Autodesk Inventor part; units mm, degrees
ref_plane "YZ Plane" through (0, 0, 0) normal (1, 0, 0) x (0, 1, 0)
ref_plane "XZ Plane" through (0, 0, 0) normal (0, 1, 0) x (-1, 0, 0)
ref_plane "XY Plane" through (0, 0, 0) normal (0, 0, 1) x (1, 0, 0)
sketch "Sketch1" plane through (0, 0, 0) normal (0, 0, 1) x (1, 0, 0)
  circle A0 centre (0, 0) radius 8.7
  arc A1 (11.985896, 6.635383) -> (-11.985896, 6.635383) centre (0, 0) ccw
  line L0 (0, 52.910691) -> (0, -52.910691) construction
  line L1 (-45, -53) -> (45, -53)
  line L2 (-45, -53) -> (-11.985896, 6.635383)
  line L3 (45, -53) -> (11.985896, 6.635383)
  line L4 (12.533127, -15) -> (23.881912, -35.5)
  line L5 (23.881912, -35.5) -> (-23.881912, -35.5)
  line L6 (-12.533127, -15) -> (12.533127, -15)
  line L7 (-23.881912, -35.5) -> (-12.533127, -15)
  circle A2 centre (0, 0) radius 8.65
  dimension "d0" = 5
  dimension "d1" = 53
  dimension "d2" = 90
  dimension "d3" = 45
  dimension "d12" = 17.5
  dimension "d13" = 15
  dimension "d15" = 10
  dimension "d16" = 10
  dimension "d41" = 17.3
sketch "Sketch1 outline for Extrusion1" plane through (0, 0, 0) normal (0, 0, 1) x (1, 0, 0)
  line L0 (-45, -53) -> (45, -53)
  line L1 (45, -53) -> (11.985896, 6.635383)
  arc A0 (11.985896, 6.635383) -> (-11.985896, 6.635383) centre (0, 0) ccw
  line L2 (-11.985896, 6.635383) -> (-45, -53)
  line L3 (12.533127, -15) -> (23.881912, -35.5)
  line L4 (23.881912, -35.5) -> (-23.881912, -35.5)
  line L5 (-23.881912, -35.5) -> (-12.533127, -15)
  line L6 (-12.533127, -15) -> (12.533127, -15)
  circle A1 centre (0, 0) radius 8.65
extrude "Extrusion1" add sketch "Sketch1 outline for Extrusion1" along normal blind 5
sketch "Sketch2" plane through (0, 0, 5) normal (0, 0, 1) x (1, 0, 0)
  line L0 (45, -53) -> (11.985896, 6.635383)
  arc A0 (11.985896, 6.635383) -> (-11.985896, 6.635383) centre (0, 0) ccw
  line L1 (-11.985896, 6.635383) -> (-45, -53)
  line L2 (-45, -53) -> (45, -53)
  line L3 (12.533127, -15) -> (23.881912, -35.5)
  line L4 (23.881912, -35.5) -> (-23.881912, -35.5)
  line L5 (-23.881912, -35.5) -> (-12.533127, -15)
  line L6 (-12.533127, -15) -> (12.533127, -15)
  line L7 (39.910172, -50) -> (9.361247, 5.182379)
  arc A1 (9.361247, 5.182379) -> (-9.361247, 5.182379) centre (0, 0) ccw
  line L8 (-9.361247, 5.182379) -> (-39.910172, -50)
  line L9 (-39.910172, -50) -> (39.910172, -50)
  line L10 (-14.301359, -12) -> (-28.97174, -38.5)
  line L11 (-28.97174, -38.5) -> (28.97174, -38.5)
  line L12 (28.97174, -38.5) -> (14.301359, -12)
  line L13 (14.301359, -12) -> (-14.301359, -12)
  circle A2 centre (0, 0) radius 8.65
  point P0 (0, 0)
  point P1 (-11.653536, 1.041678)
  point P2 (11.653536, 1.041678)
  dimension "d19" = 3
  dimension "d20" = 3
  dimension "d42" = 17.3
extrude "Extrusion2" add sketch "Sketch2" along normal blind 5 contours L2 L1 A0 L0 | L9 L8 A1 L7 | L13 L12 L11 L10
sketch "Sketch3" plane through (-45, -53, 0) normal (0, -1, 0) x (1, 0, 0)
  line L0 (45, 0) -> (45, 10) construction
  line L1 (32.466873, 10) -> (57.533127, 10) construction
  line L2 (0, 0) -> (0, 10) construction
  line L3 (0, 5) -> (90, 5) construction
  line L4 (90, 0) -> (90, 10) construction
  line L5 (33.3, 5) -> (56.7, 5) construction
  circle A0 centre (45, 5) radius 8.65
  circle A1 centre (45, 5) radius 3.5
  circle A2 centre (45, 5) radius 4.5
  circle A3 centre (77.5, 5) radius 1.7
  circle A4 centre (65, 5) radius 1.7
  circle A5 centre (12.5, 5) radius 1.7
  circle A6 centre (25, 5) radius 1.7
  point P0 (56.653536, 5)
  point P1 (33.346464, 5)
  dimension "d24" = 17.3
  dimension "d25" = 7
  dimension "d32" = 9
  dimension "d35" = 3.4
  dimension "d36" = 12.5
  dimension "d37" = 3.4
  dimension "d38" = 12.5
extrude "Extrusion3" cut sketch "Sketch3" against normal blind 5 contours A0 | A2
extrude "Extrusion4" cut sketch "Sketch3" against normal blind 43 contours A1
extrude "Extrusion5" cut sketch "Sketch3" against normal up to surface (5 mm away) from surface at -38 contours A0 | A2
extrude "Extrusion6" cut sketch "Sketch3" against normal blind 6 from surface at -38 contours A1 | A2
extrude "Extrusion7" cut sketch "Sketch3" against normal blind 13 contours A3 | A4 | A5 | A6
properties part number "96mmWheelBracket_3DPrint"
For this review, take the finished solid that the model builds, in its own axes (mm). A direction names the side the tool comes from. Coordinates: 2 decimals unless noted, no trailing zeros. Order: outer loops, then holes, each group sorted by start corner. A loop starts at its lowest first (then second) coordinate and runs counter-clockwise, first axis right, second up. Notation, with made-up numbers: (-6, 66) - (47, 66) arc R28 cw to (47, 98) - close; hole circle Ø2 at (18.5, -35.75). An arc over 180 degrees is marked (long way). Answer as a JSON object with one key per item and string values. Group by question number.
1. Clearance check with flat-ended pins moving along their axes: P1, Ø4, axis at x = 9, z = 4, coming from the +Y side; P2, Ø3, axis at x = -2.5, z = 3, coming from the -Y side; P3, Ø3, axis at x = -5.5, z = 3, coming from the +Y side; P4, Ø12, axis at x = 28.5, y = -7.5, coming from the -Z side. State where each tip first meets the part, or that it passes through.
2. We need section B-B on x = -14.5. State the section outline as (y, z) points, then the cut area to 3 significant figures.
3. The part is to be moulded in two halves that separate along X. For faces 1 (the flat face through (26, -53, 5)), 2 (the flat face through (4, -48, 5)), 3 (the cylindrical face through (21.57, -46.59, 4.35)), say which applies: pulls with the +X half, pulls with the -X half, needs draft (parallel to the pull), parting line crosses it, or undercut.
4. We need section A-A on y = -2. State the section outline as (x, z) points.
5. For faces 4 (the cylindrical face through (-18.43, -46.59, 4.35)), 5 (the flat face through (-26, -53, 5)), 6 (the flat face through (10, -15, 5)), 7 (the cylindrical face through (8.65, -12.54, 4.93)), list the 3-axis set-ups (+Z, -Z, +X, -X, +Y, -Y) from which the entire face can be reached by the end or side of a thin tool; tool diameter is ignored.
6. We need section C-C on x = 0. State the section outline as (y, z) points.
7. For probe 1 along Z at (x, y) = (0, -9.75); probe 2 along Z at (x, y) = (32.5, -42.5); probe 3 along Y at (x, z) = (0.5, 4), list the stretches that pass through material, from the lowest coordinate up.
8. We need section D-D on y = -39. State the section outline as (x, z) points, then the cut area to 3 significant figures.
Final values:
{
 "1": {"P1": "y = 11.78", "P2": "y = -48", "P3": "y = 13.1", "P4": "through"},
 "2": {"outline": "(-53, 0) - (-35.5, 0) - (-35.5, 10) - (-53, 10) - close; (-18.55, 0) - (2.09, 0) - (2.09, 10) - (-18.55, 10) - close", "area": "381 mm²"},
 "3": {"face 1": "needs draft", "face 2": "undercut", "face 3": "undercut"},
 "4": {"outline": "(-16.77, 0) - (-8.42, 0) - (-8.42, 10) - (-16.77, 10) - close; (8.42, 0) - (16.77, 0) - (16.77, 10) - (8.42, 10) - close"},
 "5": {"face 4": "-Y", "face 5": "+Z, -Z, +X, -X, -Y", "face 6": "+Z, -Z", "face 7": "none"},
 "6": {"outline": "(-48, 0) - (-35.5, 0) - (-35.5, 1.5) - (-48, 1.5) - close; (-48, 8.5) - (-35.5, 8.5) - (-35.5, 10) - (-48, 10) - close; (-10, 0) - (-8.65, 0) - (-8.65, 10) - (-10, 10) - (-10, 9.5) - (-9, 9.5) - (-9, 0.5) - (-10, 0.5) - close; (8.65, 0) - (13.7, 0) - (13.7, 10) - (8.65, 10) - close"},
 "7": {"probe 1": "0 to 0.5, 9.5 to 10", "probe 2": "0 to 3.3, 6.7 to 10", "probe 3": "-9 to -8.64, 8.64 to 13.69"},
 "8": {"outline": "(-37.25, 0) - (37.25, 0) - (37.25, 10) - (-37.25, 10) - close; hole circle Ø7 at (0, 5)", "area": "707 mm²"}
}
